Source: CAD feature listing. Evaluate the final solid. Frame: model axes, mm. A direction names the side the tool comes from. Round coordinates to 2 decimals unless told otherwise and drop trailing zeros. Write each loop counter-clockwise with the first axis right and the second up, starting at its lowest first coordinate (ties: lowest second). Pieces come first, ordered by that corner, then holes. Notation, with made-up numbers: (-35, -7) -> (-6, -7) arc R27 cw to (-6, 24) -> close; hole circle Ø3 at (71.5, 4.5). An arc over 180 degrees is marked (long way). Return JSON: item names as keys, results as strings. Group by question number.
from build123d import *

# Parameters (mm, degrees)
F0_W      = 1403.35
F0_H      = 863.6
F1_DEPTH  = 25.4
F3_DEPTH  = 25.4
F4_W      = 88.9
F4_H      = 44.45
F5_DEPTH  = 3.175
F6_W      = 88.9
F6_H      = 3.81
F7_DEPTH  = 4.445
F8_R      = 114.3
F9_W      = 88.9
F9_H      = 44.45
F10_DEPTH = 3.175
F11_W     = 12.7
F11_H     = 203.2
F12_DEPTH = 25.401
F13_R     = 9.525
F14_W     = 101.6
F14_H     = 12.7
F15_DEPTH = 25.401
F16_R     = 9.525
F17_W     = 76.2
F17_H     = 25.4
F18_DEPTH = 25.401
F19_R     = 12.69999


# Not quite as in the source:
# - a fillet or chamfer is up to 0.001 mm smaller than in the source, because OpenCascade refuses the exact size


with BuildPart() as f1:
    # F0 (on Top) → F1 (new body)
    with BuildSketch(Plane.XY):
        Rectangle(F0_W, F0_H)
    extrude(amount=F1_DEPTH)

    # F2 (on face) → F3 (cut)
    with BuildSketch(Plane.XY.offset(25.4)):
        with BuildLine():
            Line((457.2, 254), (-457.2, 254))
            ThreePointArc((-457.2, 254), (-493.1210244843, 239.1210244843), (-508, 203.2))
            Line((-508, 203.2), (-508, -203.2))
            ThreePointArc((-508, -203.2), (-493.1210244843, -239.1210244843), (-457.2, -254))
            Line((-457.2, -254), (457.2, -254))
            ThreePointArc((457.2, -254), (493.1210244843, -239.1210244843), (508, -203.2))
            Line((508, -203.2), (508, 203.2))
            ThreePointArc((508, 203.2), (493.1210244843, 239.1210244843), (457.2, 254))
        make_face()
    extrude(amount=-F3_DEPTH, mode=Mode.SUBTRACT)

    # F4 (on face) → F5 (cut)
    with BuildSketch(Plane.XY.offset(25.4)):
        with Locations((-504.825, -409.575)):
            Rectangle(F4_W, F4_H)
        with Locations((-98.425, -409.575)):
            Rectangle(F4_W, F4_H)
        with Locations((98.425, -409.575)):
            Rectangle(F4_W, F4_H)
        with Locations((504.825, -409.575)):
            Rectangle(F4_W, F4_H)
    extrude(amount=-F5_DEPTH, mode=Mode.SUBTRACT)

    # F6 (on face) → F7 (cut)
    with BuildSketch(Plane.XY.offset(25.4)):
        with Locations((-504.825, -429.895)):
            Rectangle(F6_W, F6_H)
        with Locations((-98.425, -429.895)):
            Rectangle(F6_W, F6_H)
        with Locations((98.425, -429.895)):
            Rectangle(F6_W, F6_H)
        with Locations((504.825, -429.895)):
            Rectangle(F6_W, F6_H)
    extrude(amount=-F7_DEPTH, mode=Mode.SUBTRACT)

    # F8
    f8_edges = [f1.edges().sort_by_distance(p)[0] for p in [
        (701.675, 431.8, 12.7),
        (-701.675, 431.8, 12.7),
    ]]
    fillet(f8_edges, radius=F8_R)

    # F9 (on face) → F10 (cut)
    with BuildSketch(Plane.XY.offset(25.4)):
        with Locations((98.425, 409.575)):
            Rectangle(F9_W, F9_H)
        with Locations((504.825, 409.575)):
            Rectangle(F9_W, F9_H)
        with Locations((-98.425, 409.575)):
            Rectangle(F9_W, F9_H)
        with Locations((-504.825, 409.575)):
            Rectangle(F9_W, F9_H)
    extrude(amount=-F10_DEPTH, mode=Mode.SUBTRACT)

    # F11 (on face) → F12 (cut, through all)
    with BuildSketch(Plane.XY.offset(25.4)):
        with Locations((-695.325, -228.6)):
            Rectangle(F11_W, F11_H)
        with Locations((695.325, -228.6)):
            Rectangle(F11_W, F11_H)
    extrude(amount=-F12_DEPTH, mode=Mode.SUBTRACT)

    # F13
    f13_edges = [f1.edges().sort_by_distance(p)[0] for p in [
        (-688.975, -127, 12.7),
        (-688.975, -330.2, 12.7),
        (688.975, -127, 12.7),
        (688.975, -330.2, 12.7),
    ]]
    fillet(f13_edges, radius=F13_R)

    # F14 (on face) → F15 (cut, through all)
    with BuildSketch(Plane.XY.offset(25.4)):
        with Locations((-241.3, -260.35)):
            Rectangle(F14_W, F14_H)
        with Locations((241.3, -260.35)):
            Rectangle(F14_W, F14_H)
        with Locations((-241.3, 260.35)):
            Rectangle(F14_W, F14_H)
        with Locations((241.3, 260.35)):
            Rectangle(F14_W, F14_H)
    extrude(amount=-F15_DEPTH, mode=Mode.SUBTRACT)

    # F16
    f16_edges = [f1.edges().sort_by_distance(p)[0] for p in [
        (-292.1, -266.7, 12.7),
        (190.5, -266.7, 12.7),
        (292.1, -266.7, 12.7),
        (-190.5, -266.7, 12.7),
        (190.5, 266.7, 12.7),
        (-292.1, 266.7, 12.7),
        (-190.5, 266.7, 12.7),
        (292.1, 266.7, 12.7),
    ]]
    fillet(f16_edges, radius=F16_R)

    # F17 (on face) → F18 (cut, through all)
    with BuildSketch(Plane.XY.offset(25.4)):
        with Locations((-588.01, 254)):
            Rectangle(F17_W, F17_H)
        with Locations((588.01, 254)):
            Rectangle(F17_W, F17_H)
        with Locations((588.01, -254)):
            Rectangle(F17_W, F17_H)
        with Locations((-588.01, -254)):
            Rectangle(F17_W, F17_H)
    extrude(amount=-F18_DEPTH, mode=Mode.SUBTRACT)

    # F19 (radius 12.7 in the source; OpenCascade refuses exactly that, so slightly less here)
    f19_edges = [f1.edges().sort_by_distance(p)[0] for p in [
        (-626.11, 241.3, 12.7),
        (-549.91, 241.3, 12.7),
        (-549.91, 266.7, 12.7),
        (-626.11, 266.7, 12.7),
        (-626.11, -241.3, 12.7),
        (-626.11, -266.7, 12.7),
        (-549.91, -266.7, 12.7),
        (-549.91, -241.3, 12.7),
        (626.11, -241.3, 12.7),
        (626.11, -266.7, 12.7),
        (549.91, -266.7, 12.7),
        (549.91, -241.3, 12.7),
        (549.91, 266.7, 12.7),
        (549.91, 241.3, 12.7),
        (626.11, 241.3, 12.7),
        (626.11, 266.7, 12.7),
    ]]
    fillet(f19_edges, radius=F19_R)


solid = f1.part
Item 1: Cut plane D-D on z = 14.75. Give the number of separate pieces and of enclosed holes in the cut face, and give its area (3 significant figures).
Item 2: Cut plane C-C on x = -370. Output: boundary loops of the cut face in (y, z), and give its area (3 significant figures).
Item 3: Pull-direction query (X, two-part tool) for faces 6 (the flat face through (-688.975, -230, 13)), 7 (the flat face through (-8, 431.8, 13)), 8 (the flat face through (98, -407, 22.225)); classes: +X half, -X half, draft (parallel to the pull), parting line (faces both ways), or undercut.
Item 4: Material intervals for probe 1 along X at (y, z) = (38.5, 9.5) (3 decimals); probe 2 along Y at (x, z) = (265.5, 8.25); probe 3 along Y at (x, z) = (444, 5.5), sorted ascending.
Item 5: Set-up query: faces 1 (the flat face through (-10, 294, 0)), 2 (the flat face through (98, 410, 22.225)), 3 (the cylindrical face through (492.724, -239.514, 12.878)), 4 (the flat face through (504, -407, 22.225)), 5 (the flat face through (-10, -282, 25.4)). Return all of +Z, -Z, +X, -X, +Y, -Y with unobstructed straight access to the full face (end or side cutting, diameter ignored); none if empty.
Item 6: Cut plane A-A on x = 69. Output: boundary loops of the cut face in (y, z) (3 decimals).
Item 7: First-contact query: pin 1 Ø1 at (x, z) = (102.5, 24) entering from +Y; pin 2 Ø2.5 at (x, z) = (-525.5, 24) entering from -Y; pin 3 Ø4 at (y, z) = (-311.5, 12.5) entering from +X (3 decimals). Flat tips, straight axial feed; report the tip coordinate or a pass-through.
Item 8: Cut plane B-B on y = 85.5. Output: boundary loops of the cut face in (x, z) (3 decimals).
Here are the results:
{
 "1": {"separate pieces": "1", "enclosed holes": "5", "area": "675,000 mm^2"},
 "2": {"outline": "(-431.8, 0) -> (-254, 0) -> (-254, 25.4) -> (-431.8, 25.4) -> close; (254, 0) -> (431.8, 0) -> (431.8, 25.4) -> (254, 25.4) -> close", "area": "9,030 mm^2"},
 "3": {"face 6": "-X half", "face 7": "draft", "face 8": "undercut"},
 "4": {"probe 1": "x = -701.675 to -508, 508 to 701.675", "probe 2": "y = -431.8 to -266.7, 266.7 to 431.8", "probe 3": "y = -431.8 to -254, 254 to 431.8"},
 "5": {"face 1": "-Z, +X, -X, +Y, -Y", "face 2": "+Z, +Y", "face 3": "+Z, -Z", "face 4": "+Z, -Y", "face 5": "+Z, +X, -X, +Y, -Y"},
 "6": {"outline": "(-431.8, 0) -> (-254, 0) -> (-254, 25.4) -> (-387.35, 25.4) -> (-387.35, 22.225) -> (-427.99, 22.225) -> (-427.99, 20.955) -> (-431.8, 20.955) -> close; (254, 0) -> (431.8, 0) -> (431.8, 22.225) -> (387.35, 22.225) -> (387.35, 25.4) -> (254, 25.4) -> close"},
 "7": {"pin 1": "stops at y = 387.35", "pin 2": "stops at y = -387.35", "pin 3": "stops at x = 688.975"},
 "8": {"outline": "(-701.675, 0) -> (-508, 0) -> (-508, 25.4) -> (-701.675, 25.4) -> close; (508, 0) -> (701.675, 0) -> (701.675, 25.4) -> (508, 25.4) -> close"}
}
